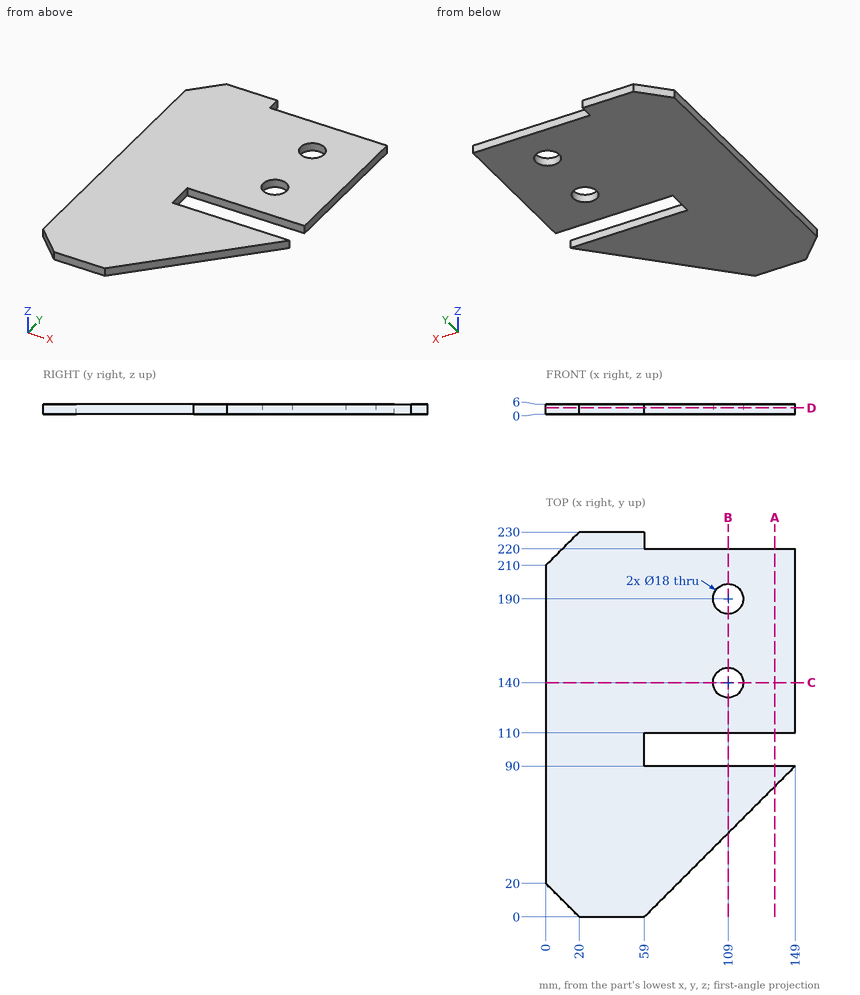
Here's the drawing with two shaded views (mm, measured from the low corner). I have some questions. Give positions to 0.01 mm unless a question says otherwise; leave off trailing zeros. Order: outer loops, then holes, each group sorted by start corner. A loop starts at its lowest first (then second) coordinate and runs counter-clockwise, first axis right, second up. Notation, with made-up numbers: (-16.5, 29.5) - (6.5, 29.5) arc R12 cw to (6.5, 40.5) - close; hole circle Ø11 at (66.25, 3.5). An arc over 180 degrees is marked (long way). Use a Markdown table: item, result. Add a question column.
Q1. If we section it at D-D on z = 3.75: Write out the boundary of the cut face in (x, y), plus the area to 3 significant figures.
Q2. If we section it at B-B on x = 109: Write out the boundary of the cut face in (y, z).
Q3. Please list where these lines run through material, in increasing order: line 1 along X through (y, z) = (140, 2.5); line 2 along Y through (x, z) = (109, 4); line 3 along Y through (x, z) = (112, 1.05).
Q4. If we section it at A-A on x = 137: Write out the boundary of the cut face in (y, z).
Q5. If we section it at C-C on y = 140: Write out the boundary of the cut face in (x, z).
Q6. I'm going to push flat-ended pins straight in: pin 1 (1.5 mm diameter, centred on y = 47, z = 1, fed in from +X); pin 2 (3 mm diameter, centred on x = 95.5, z = 3, fed in from +Y); pin 3 (14.5 mm diameter, centred on x = 109, y = 140, fed in from -Z); pin 4 (2 mm diameter, centred on y = 67, z = 3, fed in from +X). Where does each tip first touch, or does it pass through?
Answers follow:
| question | item | result |
|---|---|---|
| 1 | outline | (0, 20) - (20, 0) - (59, 0) - (149, 90) - (59, 90) - (59, 110) - (149, 110) - (149, 220) - (59, 220) - (59, 230) - (20, 230) - (0, 210) - close; hole circle Ø18 at (109, 140); hole circle Ø18 at (109, 190) |
| 1 | area | 26,600 mm^2 |
| 2 | outline | (50, 0) - (90, 0) - (90, 6) - (50, 6) - close; (110, 0) - (131, 0) - (131, 6) - (110, 6) - close; (149, 0) - (181, 0) - (181, 6) - (149, 6) - close; (199, 0) - (220, 0) - (220, 6) - (199, 6) - close |
| 3 | line 1 | x = 0 to 100, 118 to 149 |
| 3 | line 2 | y = 50 to 90, 110 to 131, 149 to 181, 199 to 220 |
| 3 | line 3 | y = 53 to 90, 110 to 131.51, 148.49 to 181.51, 198.49 to 220 |
| 4 | outline | (78, 0) - (90, 0) - (90, 6) - (78, 6) - close; (110, 0) - (220, 0) - (220, 6) - (110, 6) - close |
| 5 | outline | (0, 0) - (100, 0) - (100, 6) - (0, 6) - close; (118, 0) - (149, 0) - (149, 6) - (118, 6) - close |
| 6 | pin 1 | stops at x = 106.75 |
| 6 | pin 2 | stops at y = 220 |
| 6 | pin 3 | passes through |
| 6 | pin 4 | stops at x = 127 |
